The drawing under review shows one solid part. Ordinate dimensions are in mm from its lowest x, y, z. Coordinates: 2 decimals unless noted, no trailing zeros. Write each loop counter-clockwise with the first axis right and the second up, starting at its lowest first coordinate (ties: lowest second). Pieces come first, ordered by that corner, then holes.
Q1. Take a section at A-A (y = 10). Give the boundary of the cut face in (x, z), and give its area (3 significant figures).
Q2. Take a section at C-C (x = 20). Give the boundary of the cut face in (y, z), and give its area (3 significant figures).
Q3. For probe 1 along Y at (x, z) = (8, 4.7); probe 2 along X at (y, z) = (10, 4.8); probe 3 along Y at (x, z) = (20, 4.1), list the stretches that pass through material, from the lowest coordinate up.
Q4. Take a section at B-B (z = 4.6). Give the boundary of the cut face in (x, y), and give its area (3 significant figures).
Q5. Mouldability with a two-part tool opening along X and no side actions: class the marked faces 1, 2 and 3 as pulls with the +X half, pulls with the -X half, needs draft (parallel to the pull), parting line crosses it, or undercut.
Q6. Take a section at D-D (y = 35). Give the boundary of the cut face in (x, z), and give its area (3 significant figures).
Q7. Insertion check: pin 1 (6.5 mm diameter, centred on x = 32, y = 10, fed in from +Z); pin 2 (17.5 mm diameter, centred on x = 20, y = 35, fed in from -Z). Each pin has a flat end and moves straight along its axis. Give the tip position at first contact, or say it passes through.
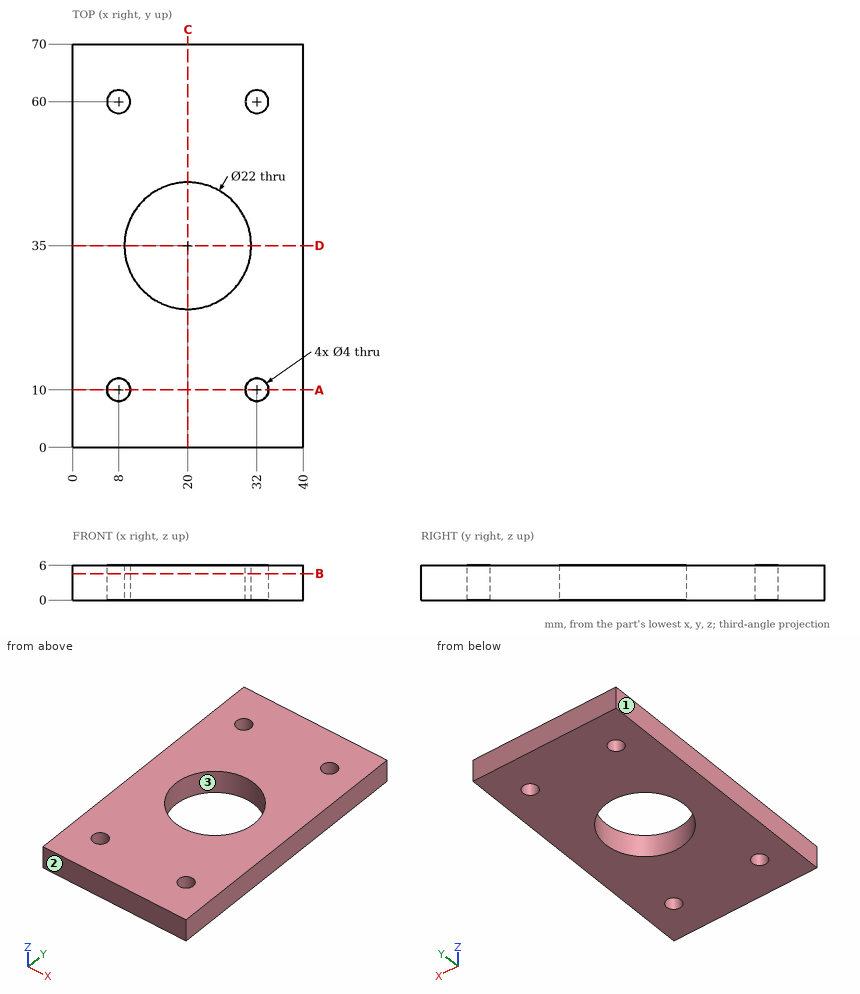
Response:
1. outline: (0, 0) - (6, 0) - (6, 6) - (0, 6) - close; (10, 0) - (30, 0) - (30, 6) - (10, 6) - close; (34, 0) - (40, 0) - (40, 6) - (34, 6) - close
1. area: 192 mm2
2. outline: (0, 0) - (24, 0) - (24, 6) - (0, 6) - close; (46, 0) - (70, 0) - (70, 6) - (46, 6) - close
2. area: 288 mm2
3. probe 1: y = 0 to 8, 12 to 58, 62 to 70
3. probe 2: x = 0 to 6, 10 to 30, 34 to 40
3. probe 3: y = 0 to 24, 46 to 70
4. outline: (0, 0) - (40, 0) - (40, 70) - (0, 70) - close; hole circle Ø4 at (8, 10); hole circle Ø4 at (8, 60); hole circle Ø22 at (20, 35); hole circle Ø4 at (32, 10); hole circle Ø4 at (32, 60)
4. area: 2,370 mm2
5. face 1: pulls with the -X half
5. face 2: needs draft
5. face 3: undercut
6. outline: (0, 0) - (9, 0) - (9, 6) - (0, 6) - close; (31, 0) - (40, 0) - (40, 6) - (31, 6) - close
6. area: 108 mm2
7. pin 1: stops at z = 6
7. pin 2: passes through
